For this review, take the finished solid that the model builds, in its own axes (mm). Face numbers are marked on the shaded views. A direction names the side the tool comes from. Give positions to 0.01 mm unless a question says otherwise; leave off trailing zeros. Write each loop counter-clockwise with the first axis right and the second up, starting at its lowest first coordinate (ties: lowest second). Pieces come first, ordered by that corner, then holes.
from build123d import *

# Parameters (mm, degrees)
F0_W      = 60.5
F0_H      = 40.64
F1_DEPTH  = 12.7
F2_W      = 64.6999999881
F2_H      = 44.1999999881
F2_W_2    = 61.5
F2_H_2    = 41
F3_DEPTH  = 11
F4_DEPTH  = 1.6
F5_DEPTH  = 8.8
F6_W      = 0.5
F6_H      = 35
F7_DEPTH  = 16
F8_DEPTH  = 60.7
F9_R      = 2.5
F10_R     = 2.5
F11_W     = 8
F11_H     = 5
F12_DEPTH = 1.71


# Not quite as in the source:
# - a feature names something its author has since deleted; it is built from what else it names


with BuildPart() as f1:
    # F0 (on Top) → F1 (new body)
    with BuildSketch(Plane.XY):
        Rectangle(F0_W, F0_H)
    extrude(amount=F1_DEPTH)



with BuildPart() as f3:
    # F2 (on Top) → F3 (new body)
    with BuildSketch(Plane.XY):
        Rectangle(F2_W, F2_H)
        Rectangle(F2_W_2, F2_H_2, mode=Mode.SUBTRACT)
    extrude(amount=F3_DEPTH)


with BuildPart() as f1_1:
    add(f1.part)

    add(f3.part)  # F4 merges F3
    # F2 (on Top) → F4 (join)
    with BuildSketch(Plane.XY):
        Rectangle(F2_W_2, F2_H_2)
    extrude(amount=F4_DEPTH)

    # F5 (cut): a face of the model
    f5_faces = [f1_1.faces().sort_by_distance(p)[0] for p in [
        (-30.25, 0, 7.15),
    ]]
    extrude(f5_faces, amount=F5_DEPTH, mode=Mode.SUBTRACT)

    # F6 (on face) → F7 (cut)
    with BuildSketch(Plane(origin=(0, 0, 0), x_dir=(1, 0, 0), z_dir=(0, 0, -1))):
        with Locations((22, 0)):
            Rectangle(F6_W, F6_H)
        with Locations((16.5, 0)):
            Rectangle(F6_W, F6_H)
        with Locations((11, 0)):
            Rectangle(F6_W, F6_H)
        with Locations((5.5, 0)):
            Rectangle(F6_W, F6_H)
        Rectangle(F6_W, F6_H)
    extrude(amount=-F7_DEPTH, mode=Mode.SUBTRACT)

    # F8 (cut): a face of the model
    f8_faces = [f1_1.faces().sort_by_distance(p)[0] for p in [
        (-30.25, 0, 7.15),
    ]]
    extrude(f8_faces, amount=-F8_DEPTH, mode=Mode.SUBTRACT)

    # F9
    f9_edges = [f1_1.edges().sort_by_distance(p)[0] for p in [
        (32.35, 22.1, 5.5),
        (32.35, -22.1, 5.5),
    ]]
    fillet(f9_edges, radius=F9_R)

    # F10
    f10_edges = [f1_1.edges().sort_by_distance(p)[0] for p in [
        (-32.35, 22.1, 5.5),
        (-32.35, -22.1, 5.5),
    ]]
    fillet(f10_edges, radius=F10_R)

    # F14: F12 across plane


with BuildPart() as f12:
    # F11 (on face) → F12 (new body)
    with BuildSketch(Plane.YZ.offset(32.349999994)):
        with Locations((13.1696772724, 8.5)):
            Rectangle(F11_W, F11_H)
    extrude(amount=-F12_DEPTH)


with BuildPart() as f1_2:
    add(f1_1.part)
    add(f12.part.mirror(Plane(origin=(0, 0, 5.5), x_dir=(-1, 0, 0), z_dir=(0, 1, 0))), mode=Mode.SUBTRACT)


solid = f1_2.part
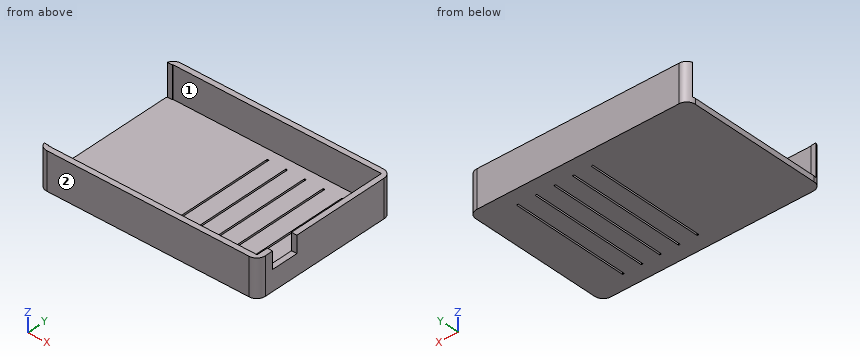
(1) We need section C-C (z = 3.5). Write out the cut boundary in (x, y), and give its area (3 significant figures).
(2) Tool access review of the marked faces 1 and 2: name each direction out of +Z, -Z, +X, -X, +Y, -Y from which nothing blocks a thin tool from reaching the whole face with its end or side.
(3) For L1, parallel to Y at x = 9.5, z = 8.25; L2, parallel to Z at x = 29, y = -15.5; L3, parallel to X at y = 2.5, z = 7.25, list the stretches that pass through material, from the lowest coordinate up.
(4) We need section B-B (z = 8.25). Write out the cut boundary in (x, y), and give its area (3 significant figures).
(5) Clearance check with flat-ended pins moving along their axes: pin 1 Ø4 at (y, z) = (-13.5, 6) entering from -X; pin 2 Ø10 at (x, y) = (24.5, -3) entering from +Z. State where each tip first meets the part, or that it passes through.
(6) We need section D-D (y = -16). Write out the cut boundary in (x, z), and give its area (3 significant figures).
(7) We need section A-A (y = -5). Write out the cut boundary in (x, z), and give its area (3 significant figures).
The answers:
1. outline: (-32.24, -20.32) arc R2.5 ccw to (-29.85, -22.1) - (29.85, -22.1) arc R2.5 ccw to (32.35, -19.6) - (32.35, 19.6) arc R2.5 ccw to (29.85, 22.1) - (-29.85, 22.1) arc R2.5 ccw to (-32.24, 20.32) - (-30.75, 20.32) - (-30.75, 20.5) - (30.75, 20.5) - (30.75, -20.5) - (-30.75, -20.5) - (-30.75, -20.32) - close
1. area: 268 mm2
2. face 1: +Z
2. face 2: +Z, -Z, +X, -X, -Y
3. L1: y = -22.1 to -20.5, 20.5 to 22.1
3. L2: z = 0 to 1.6
3. L3: x = 30.75 to 32.35
4. outline: (-32.24, -20.32) arc R2.5 ccw to (-29.85, -22.1) - (29.85, -22.1) arc R2.5 ccw to (32.35, -19.6) - (32.35, -17.17) - (30.75, -17.17) - (30.75, -20.5) - (-30.75, -20.5) - (-30.75, -20.32) - close; (-32.24, 20.32) - (-30.75, 20.32) - (-30.75, 20.5) - (30.75, 20.5) - (30.75, -9.17) - (32.35, -9.17) - (32.35, 19.6) arc R2.5 ccw to (29.85, 22.1) - (-29.85, 22.1) arc R2.5 ccw to start
4. area: 255 mm2
5. pin 1: stops at x = 30.75
5. pin 2: stops at z = 1.6
6. outline: (-32.35, 0) - (-0.25, 0) - (-0.25, 1.6) - (-32.35, 1.6) - close; (0.25, 0) - (5.25, 0) - (5.25, 1.6) - (0.25, 1.6) - close; (5.75, 0) - (10.75, 0) - (10.75, 1.6) - (5.75, 1.6) - close; (11.25, 0) - (16.25, 0) - (16.25, 1.6) - (11.25, 1.6) - close; (16.75, 0) - (21.75, 0) - (21.75, 1.6) - (16.75, 1.6) - close; (22.25, 0) - (32.35, 0) - (32.35, 6) - (30.75, 6) - (30.75, 1.6) - (22.25, 1.6) - close
6. area: 107 mm2
7. outline: (-32.35, 0) - (-0.25, 0) - (-0.25, 1.6) - (-32.35, 1.6) - close; (0.25, 0) - (5.25, 0) - (5.25, 1.6) - (0.25, 1.6) - close; (5.75, 0) - (10.75, 0) - (10.75, 1.6) - (5.75, 1.6) - close; (11.25, 0) - (16.25, 0) - (16.25, 1.6) - (11.25, 1.6) - close; (16.75, 0) - (21.75, 0) - (21.75, 1.6) - (16.75, 1.6) - close; (22.25, 0) - (32.35, 0) - (32.35, 11) - (30.75, 11) - (30.75, 1.6) - (22.25, 1.6) - close
7. area: 115 mm2
